from build123d import *

# Parameters (mm, degrees)
F2_R     = 1
F3_DEPTH = 48.006


# Not quite as in the source:
# - the program builds the solid bodies; features that only make, move or delete a surface that nothing else refers to are left out


with BuildPart() as f1:
    # F0 (on Front) → F1 (revolve)
    with BuildSketch(Plane.XZ):
        Polygon((-48.5, 6.5), (-49.5, 6.5), (-49.5, -6.5), (-48.5, -6.5), (-48.5, -1.5), (-45.5, -1.5), (-45.5, 0), (-45.5, 1.5), (-48.5, 1.5), align=None)
    revolve(axis=Axis((0, 0, -3.8321989188), (0, 0, -1)))

    # F2 (on Right) → F3 (cut)
    with BuildSketch(Plane.YZ):
        with Locations((-3, 0)):
            Circle(F2_R)
        with BuildLine():
            ThreePointArc((4, 0), (3, 1), (2, 0))
            ThreePointArc((2, 0), (3, -1), (4, 0))
        make_face()
    extrude(amount=F3_DEPTH, mode=Mode.SUBTRACT)


solid = f1.part
Could you check a few things on this model? Use its own coordinates, in mm. A direction names the side the tool comes from. Give positions to 0.01 mm unless a question says otherwise; leave off trailing zeros. Order: outer loops, then holes, each group sorted by start corner. A loop starts at its lowest first (then second) coordinate and runs counter-clockwise, first axis right, second up.
1. For faces 1 (the cylindrical face through (-22.38, -43.028, -3.965)), 2 (the flat face through (33, -36, 6.5)), 3 (the cylindrical face through (-22.38, -43.028, 4.035)), which set-ups out of +Z, -Z, +X, -X, +Y, -Y let a thin tool reach every point of the face, with its end or its side?
2. Suppose I cut it at A-A (x = 0). List the corners of the cut face in (y, z) for me, plus the area to 3 significant figures.
3. Suppose I cut it at B-B (y = 43). List the corners of the cut face in (x, z) for me, plus the area to 3 significant figures.
4. Will these pins go through, and if not, where does the flat tip stop? P1, Ø2.5, axis at y = 3, z = 0, coming from the +X side; P2, Ø2, axis at x = -18.5, z = 1, coming from the -Y side; P3, Ø3, axis at y = 18.5, z = -5, coming from the -X side; P4, Ø4, axis at x = -33, y = -26.5, coming from the +Z side.
5. I need wall thicknesses on L1, parallel to Y at x = 0, z = -0.75; L2, parallel to Y at x = 0, z = -2.7; L3, parallel to Z at x = 47.35, y = -3. Which ranges of each line are inside material? Lowest first, please.
6. We'd pull the mould along Y, two halves only. Please class faces 4 (the cylindrical face through (-43.4, 13.67, 0.02)), 5 (the cylindrical face through (6.44, 49.08, -0.09)), 6 (the flat face through (-33, -36, -6.5)): pulls with the +Y half, pulls with the -Y half, needs draft (parallel to the pull), parting line crosses it, or undercut.
Solved:
1. face 1: -Z
1. face 2: +Z, +X, -X, +Y, -Y
1. face 3: +Z
2. outline: (-49.5, -6.5) - (-48.5, -6.5) - (-48.5, -1.5) - (-45.5, -1.5) - (-45.5, 1.5) - (-48.5, 1.5) - (-48.5, 6.5) - (-49.5, 6.5) - close; (45.5, -1.5) - (48.5, -1.5) - (48.5, -6.5) - (49.5, -6.5) - (49.5, 6.5) - (48.5, 6.5) - (48.5, 1.5) - (45.5, 1.5) - close
2. area: 44.0 mm2
3. outline: (-24.52, -6.5) - (-22.43, -6.5) - (-22.43, -1.5) - (-14.87, -1.5) - (-14.87, 1.5) - (-22.43, 1.5) - (-22.43, 6.5) - (-24.52, 6.5) - close; (14.87, -1.5) - (22.43, -1.5) - (22.43, -6.5) - (24.52, -6.5) - (24.52, 6.5) - (22.43, 6.5) - (22.43, 1.5) - (14.87, 1.5) - close
3. area: 99.6 mm2
4. P1: stops at x = 49.47
4. P2: stops at y = -46.3
4. P3: stops at x = -46.49
4. P4: passes through
5. L1: y = -49.5 to -45.5, 45.5 to 49.5
5. L2: y = -49.5 to -48.5, 48.5 to 49.5
5. L3: z = -1.5 to -1, 1 to 1.5
6. face 4: undercut
6. face 5: parting line crosses it
6. face 6: needs draft
